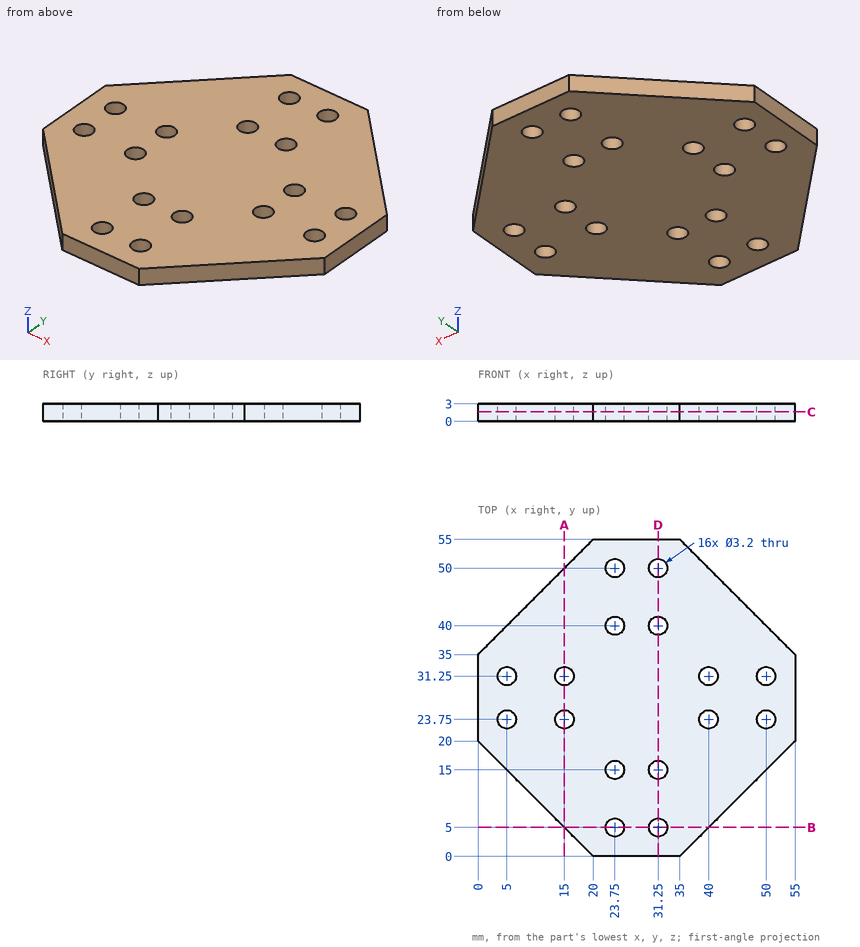
Could you check a few things on this drawing? It's one solid part, dimensions in mm from its lowest x, y, z. Coordinates: 2 decimals unless noted, no trailing zeros. Write each loop counter-clockwise with the first axis right and the second up, starting at its lowest first coordinate (ties: lowest second). Pieces come first, ordered by that corner, then holes. Notation, with made-up numbers: (-34.5, 16) - (3.5, 16) arc R7 cw to (3.5, 20) - close; hole circle Ø8 at (1.5, 19.25). An arc over 180 degrees is marked (long way). Return JSON: item names as keys, results as strings. Group by question number.
Item 1: Please list where these lines run through material, in increasing order: probe 1 along Y at (x, z) = (31.25, 1.75); probe 2 along Y at (x, z) = (40, 2.2); probe 3 along Y at (x, z) = (5, 2.15).
Item 2: If we section it at B-B (y = 5): Write out the boundary of the cut face in (x, z), then the cut area to 3 significant figures.
Item 3: If we section it at C-C (z = 1.65): Count the separate pieces of the cut face and the enclosed holes in it, then the cut area to 3 significant figures.
Item 4: I'm going to push flat-ended pins straight in: pin 1 Ø3 at (x, y) = (5, 23.75) entering from +Z; pin 2 Ø6 at (x, y) = (31, 31) entering from -Z. Where does each tip first touch, or does it pass through?
Item 5: If we section it at A-A (x = 15): Write out the boundary of the cut face in (y, z), then the cut area to 3 significant figures.
Item 6: If we section it at D-D (x = 31.25): Write out the boundary of the cut face in (y, z).
Return value:
{
 "1": {"probe 1": "y = 0 to 3.4, 6.6 to 13.4, 16.6 to 38.4, 41.6 to 48.4, 51.6 to 55", "probe 2": "y = 5 to 22.15, 25.35 to 29.65, 32.85 to 50", "probe 3": "y = 15 to 22.15, 25.35 to 29.65, 32.85 to 40"},
 "2": {"outline": "(15, 0) - (22.15, 0) - (22.15, 3) - (15, 3) - close; (25.35, 0) - (29.65, 0) - (29.65, 3) - (25.35, 3) - close; (32.85, 0) - (40, 0) - (40, 3) - (32.85, 3) - close", "area": "55.8 mm^2"},
 "3": {"separate pieces": "1", "enclosed holes": "16", "area": "2,100 mm^2"},
 "4": {"pin 1": "passes through", "pin 2": "stops at z = 0"},
 "5": {"outline": "(5, 0) - (22.15, 0) - (22.15, 3) - (5, 3) - close; (25.35, 0) - (29.65, 0) - (29.65, 3) - (25.35, 3) - close; (32.85, 0) - (50, 0) - (50, 3) - (32.85, 3) - close", "area": "116 mm^2"},
 "6": {"outline": "(0, 0) - (3.4, 0) - (3.4, 3) - (0, 3) - close; (6.6, 0) - (13.4, 0) - (13.4, 3) - (6.6, 3) - close; (16.6, 0) - (38.4, 0) - (38.4, 3) - (16.6, 3) - close; (41.6, 0) - (48.4, 0) - (48.4, 3) - (41.6, 3) - close; (51.6, 0) - (55, 0) - (55, 3) - (51.6, 3) - close"}
}
